from build123d import *

# Parameters (mm, degrees)
SKETCH_1_W          = 32.5
SKETCH_1_H          = 7
EXTRUDE_1_DEPTH     = 21
CUT_EXTRUDE_1_REACH = 28.783
SKETCH_2_R          = 1.35
CUT_EXTRUDE_2_REACH = 29.46


with BuildPart() as part:
    # 草图1 → 凸台-拉伸1 (new body)
    with BuildSketch(Plane(origin=(0, 0, 0), x_dir=(1, 0, 0), z_dir=(0, 1, 0))):
        Rectangle(SKETCH_1_W, SKETCH_1_H)
    extrude(amount=EXTRUDE_1_DEPTH)

    # 草图2 → 切除-拉伸1 (cut, up to next)
    with BuildSketch(Plane.XZ, mode=Mode.PRIVATE) as cut_extrude_1_sk1:
        with Locations(Location((-10, 0, 0), (0, 0, 270))):
            Circle(SKETCH_2_R)
    cut_extrude_1_tool1 = extrude(cut_extrude_1_sk1.sketch, amount=-CUT_EXTRUDE_1_REACH, mode=Mode.PRIVATE) & part.part
    # 草图2 → 切除-拉伸1 (cut, up to next)
    with BuildSketch(Plane.XZ, mode=Mode.PRIVATE) as cut_extrude_1_sk2:
        with Locations(Location((10, 0, 0), (0, 0, 270))):
            Circle(SKETCH_2_R)
    cut_extrude_1_tool2 = extrude(cut_extrude_1_sk2.sketch, amount=-CUT_EXTRUDE_1_REACH, mode=Mode.PRIVATE) & part.part
    add(cut_extrude_1_tool1.solids().sort_by_distance((-10, 0, 0))[0], mode=Mode.SUBTRACT)
    add(cut_extrude_1_tool2.solids().sort_by_distance((10, 0, 0))[0], mode=Mode.SUBTRACT)

    # 草图3 → 切除-拉伸2 (cut, up to next)
    with BuildSketch(Plane.XY.offset(3.5), mode=Mode.PRIVATE) as cut_extrude_2_sk1:
        Polygon((-16.25, 21), (-16.25, 7), (16.25, 21), align=None)
    cut_extrude_2_tool1 = extrude(cut_extrude_2_sk1.sketch, amount=-CUT_EXTRUDE_2_REACH, mode=Mode.PRIVATE) & part.part
    add(cut_extrude_2_tool1.solids().sort_by_distance((-5.416667, 16.333333, 3.5))[0], mode=Mode.SUBTRACT)

    # 切除-扫描1: sweep along a path in 草图5
    with BuildLine(Plane(origin=(-5.086843681, 11.80874426, 0), x_dir=(0.9184126158110062, 0.3956238960416641, 0), z_dir=(-0.3956238960416641, 0.9184126158110062, 0))) as sweep_1_path:
        Line((-12.154837735, 0), (23.232306824, 0))
    # 草图4 → 切除-扫描1 (sweep, cut)
    with BuildSketch(Plane.ZY.offset(16.25)):
        with BuildLine():
            Line((-2, 7), (2, 7))
            ThreePointArc((2, 7), (0, 5), (-2, 7))
        make_face()
    sweep(path=sweep_1_path.line, mode=Mode.SUBTRACT)


solid = part.part
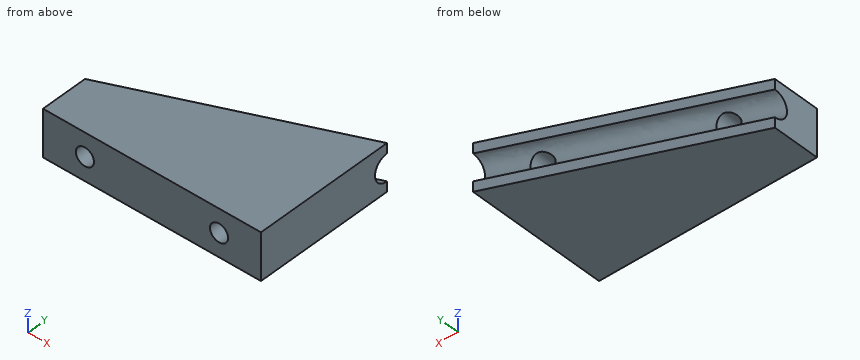
The model under review builds one solid part; all positions refer to its coordinate system, in mm. Give positions to 0.01 mm unless a question says otherwise; leave off trailing zeros. Order: outer loops, then holes, each group sorted by start corner. A loop starts at its lowest first (then second) coordinate and runs counter-clockwise, first axis right, second up. Notation, with made-up numbers: M 10.5,84.25 L 48.5,84.25 A10 ccw 48.5,94.25 Z; hole C 41.25,-7 d9. An arc over 180 degrees is marked long. One line per question, with ' | ' between items. Start each with the question number.
1) Consider section B-B, the plane z = -0.25. State how many separate pieces and enclosed holes the cut face has, then the cut area to 3 significant figures.
2) Clearance check with flat-ended pins moving along their axes: P1, Ø3, axis at x = 10, z = 0, coming from the +Y side; P2, Ø2, axis at x = -10, z = 0, coming from the -Y side. State where each tip first meets the part, or that it passes through.
3) Consider section A-A, the plane y = 2. Give the boundary of the cut face in (x, z).
4) Wall thickness on L1, parallel to Z at x = 10, y = 11; L2, parallel to X at y = 6.5, z = 0; L3, parallel to X at y = 7, z = 0.75: over which ranges is each line inside the solid? List them lowest first. Write a range as from..to.
5) Consider section C-C, the plane z = -3. Give the boundary of the cut face in (x, y), then the cut area to 3 significant figures.
Found:
1) separate pieces: 3 | enclosed holes: 0 | area: 327 mm²
2) P1: stops at y = 17.11 | P2: passes through
3) outline: M -16.25,-3.5 L 16.25,-3.5 L 16.25,3.5 L -16.25,3.5 Z; hole C -10,0 d2.7; hole C 10,0 d2.7
4) L1: z = -3.5..-1.35, 1.35..3.5 | L2: x = -12.77..-11.35, -8.65..8.65, 11.35..16.25 | L3: x = -11.95..-11.12, -8.88..8.88, 11.12..16.25
5) outline: M -16.25,0 L 16.25,0 L 16.25,21 L -16.25,7 Z | area: 455 mm²
